```python
from build123d import *

# Parameters (mm, degrees)
SKETCH1_3_W         = 27.034600944
SKETCH1_3_H         = 64.50289226
BOSS_EXTRUDE2_DEPTH = 2
SKETCH1_4_W         = 27.034600944
SKETCH1_4_H         = 64.50289226
SKETCH1_4_R         = 2.5
SKETCH1_4_W_2       = 18.5
SKETCH1_4_H_2       = 23
SKETCH1_4_R_2       = 0.75
BOSS_EXTRUDE3_DEPTH = 3
SKETCH1_R           = 2.5
SKETCH1_R_2         = 0.75
BOSS_EXTRUDE6_DEPTH = 12
CUT_EXTRUDE1_START  = -3
SKETCH2_W           = 10.1
SKETCH2_H           = 7
SKETCH2_H_2         = 5.610263073
CUT_EXTRUDE1_DEPTH  = 3.5
BOSS_EXTRUDE7_DEPTH = 18.5
SKETCH5_W           = 27.034600944
SKETCH5_H           = 64.50289226
SKETCH5_W_2         = 23.034600944
SKETCH5_H_2         = 59.50289226
BOSS_EXTRUDE9_DEPTH = 29
SKETCH6_W           = 23.034600944
SKETCH6_H           = 1
CUT_EXTRUDE2_DEPTH  = 0.5
CUT_EXTRUDE3_REACH  = 75.262
SKETCH8_W           = 14.7
SKETCH8_H           = 8.1
CUT_EXTRUDE4_REACH  = 64.464
SKETCH9_W           = 6.5
SKETCH9_H           = 15.5
SKETCH11_W          = 10.1
SKETCH11_H          = 2
CUT_EXTRUDE5_DEPTH  = 0.5


with BuildPart() as part:
    # Sketch1<3> → Boss-Extrude2 (new body)
    with BuildSketch(Plane.XY):
        with Locations((0, 14.082400554)):
            Rectangle(SKETCH1_3_W, SKETCH1_3_H)
    extrude(amount=BOSS_EXTRUDE2_DEPTH)

    # Sketch1<4> → Boss-Extrude3 (add)
    # profile 1 of 15: a face of its own
    with BuildSketch(Plane.XY):
        with Locations((0, 14.082400554)):
            Rectangle(SKETCH1_4_W, SKETCH1_4_H)
        with Locations((-8.75, -8.667715428)):
            Circle(SKETCH1_4_R, mode=Mode.SUBTRACT)
        with Locations((8.75, -8.667715428)):
            Circle(SKETCH1_4_R, mode=Mode.SUBTRACT)
        with Locations((8.75, 13.832284572)):
            Circle(SKETCH1_4_R, mode=Mode.SUBTRACT)
        with Locations((-8.75, 13.832284572)):
            Circle(SKETCH1_4_R, mode=Mode.SUBTRACT)
        with Locations((0, 32.833846684)):
            Rectangle(SKETCH1_4_W_2, SKETCH1_4_H_2, mode=Mode.SUBTRACT)
    # profile 2 of 15: a face of its own
    with BuildSketch(Plane.XY):
        with Locations((8.75, 13.832284572)):
            Circle(SKETCH1_4_R)
        with Locations((8.75, 13.832284572)):
            Circle(SKETCH1_4_R_2, mode=Mode.SUBTRACT)
    # profile 3 of 15: a face of its own
    with BuildSketch(Plane.XY):
        with Locations((8.75, 13.832284572)):
            Circle(SKETCH1_4_R_2)
    # profile 4 of 15: a face of its own
    with BuildSketch(Plane.XY):
        with Locations((-8.75, 13.832284572)):
            Circle(SKETCH1_4_R)
        with Locations((-8.75, 13.832284572)):
            Circle(SKETCH1_4_R_2, mode=Mode.SUBTRACT)
    # profile 5 of 15: a face of its own
    with BuildSketch(Plane.XY):
        with Locations((-8.75, 13.832284572)):
            Circle(SKETCH1_4_R_2)
    # profile 6 of 15: a face of its own
    with BuildSketch(Plane.XY):
        with BuildLine():
            ThreePointArc((-6.278285008, -8.292715428), (-8.75, -6.167715428), (-11.221714992, -8.292715428))
            Line((-11.221714992, -8.292715428), (-9.399519053, -8.292715428))
            ThreePointArc((-9.399519053, -8.292715428), (-8.75, -7.917715428), (-8.100480947, -8.292715428))
            Line((-8.100480947, -8.292715428), (-6.278285008, -8.292715428))
        make_face()
    # profile 7 of 15: a face of its own
    with BuildSketch(Plane.XY):
        with BuildLine():
            Line((-9.399519053, -8.292715428), (-11.221714992, -8.292715428))
            ThreePointArc((-11.221714992, -8.292715428), (-8.938032605, -11.160634147), (-6.25, -8.667715428))
            ThreePointArc((-6.25, -8.667715428), (-6.257081281, -8.479682824), (-6.278285008, -8.292715428))
            Line((-6.278285008, -8.292715428), (-8.100480947, -8.292715428))
            ThreePointArc((-8.100480947, -8.292715428), (-8.02555563, -8.473601145), (-8, -8.667715428))
            ThreePointArc((-8, -8.667715428), (-8.944114284, -9.392159798), (-9.399519053, -8.292715428))
        make_face()
    # profile 8 of 15: a face of its own
    with BuildSketch(Plane.XY):
        with BuildLine():
            ThreePointArc((-8.100480947, -8.292715428), (-8.75, -7.917715428), (-9.399519053, -8.292715428))
            Line((-9.399519053, -8.292715428), (-8.100480947, -8.292715428))
        make_face()
    # profile 9 of 15: a face of its own
    with BuildSketch(Plane.XY):
        with BuildLine():
            Line((-8.100480947, -8.292715428), (-9.399519053, -8.292715428))
            ThreePointArc((-9.399519053, -8.292715428), (-8.944114284, -9.392159798), (-8, -8.667715428))
            ThreePointArc((-8, -8.667715428), (-8.02555563, -8.473601145), (-8.100480947, -8.292715428))
        make_face()
    # profile 10 of 15: a face of its own
    with BuildSketch(Plane.XY):
        with BuildLine():
            ThreePointArc((-6.278285008, -8.292715428), (-8.75, -6.167715428), (-11.221714992, -8.292715428))
            Line((-11.221714992, -8.292715428), (-9.399519053, -8.292715428))
            ThreePointArc((-9.399519053, -8.292715428), (-8.75, -7.917715428), (-8.100480947, -8.292715428))
            Line((-8.100480947, -8.292715428), (-6.278285008, -8.292715428))
        make_face()
    # profile 11 of 15: a face of its own
    with BuildSketch(Plane.XY):
        with BuildLine():
            Line((-9.399519053, -8.292715428), (-11.221714992, -8.292715428))
            ThreePointArc((-11.221714992, -8.292715428), (-8.938032605, -11.160634147), (-6.25, -8.667715428))
            ThreePointArc((-6.25, -8.667715428), (-6.257081281, -8.479682824), (-6.278285008, -8.292715428))
            Line((-6.278285008, -8.292715428), (-8.100480947, -8.292715428))
            ThreePointArc((-8.100480947, -8.292715428), (-8.02555563, -8.473601145), (-8, -8.667715428))
            ThreePointArc((-8, -8.667715428), (-8.944114284, -9.392159798), (-9.399519053, -8.292715428))
        make_face()
    # profile 12 of 15: a face of its own
    with BuildSketch(Plane.XY):
        with BuildLine():
            ThreePointArc((-8.100480947, -8.292715428), (-8.75, -7.917715428), (-9.399519053, -8.292715428))
            Line((-9.399519053, -8.292715428), (-8.100480947, -8.292715428))
        make_face()
    # profile 13 of 15: a face of its own
    with BuildSketch(Plane.XY):
        with BuildLine():
            Line((-8.100480947, -8.292715428), (-9.399519053, -8.292715428))
            ThreePointArc((-9.399519053, -8.292715428), (-8.944114284, -9.392159798), (-8, -8.667715428))
            ThreePointArc((-8, -8.667715428), (-8.02555563, -8.473601145), (-8.100480947, -8.292715428))
        make_face()
    # profile 14 of 15: a face of its own
    with BuildSketch(Plane.XY):
        with Locations((8.75, -8.667715428)):
            Circle(SKETCH1_4_R)
        with Locations((8.75, -8.667715428)):
            Circle(SKETCH1_4_R_2, mode=Mode.SUBTRACT)
    # profile 15 of 15: a face of its own
    with BuildSketch(Plane.XY):
        with Locations((8.75, -8.667715428)):
            Circle(SKETCH1_4_R_2)
    extrude(amount=-BOSS_EXTRUDE3_DEPTH)

    # Sketch1 → Boss-Extrude6 (add)
    # profile 1 of 4: a face of its own
    with BuildSketch(Plane.XY):
        with BuildLine():
            Line((-9.399519053, -8.292715428), (-11.221714992, -8.292715428))
            ThreePointArc((-11.221714992, -8.292715428), (-8.75, -11.167715428), (-6.278285008, -8.292715428))
            Line((-6.278285008, -8.292715428), (-8.100480947, -8.292715428))
            ThreePointArc((-8.100480947, -8.292715428), (-8.75, -9.417715428), (-9.399519053, -8.292715428))
        make_face()
    # profile 2 of 4: a face of its own
    with BuildSketch(Plane.XY):
        with Locations((-8.75, 13.832284572)):
            Circle(SKETCH1_R)
        with Locations((-8.75, 13.832284572)):
            Circle(SKETCH1_R_2, mode=Mode.SUBTRACT)
    # profile 3 of 4: a face of its own
    with BuildSketch(Plane.XY):
        with Locations((8.75, 13.832284572)):
            Circle(SKETCH1_R)
        with Locations((8.75, 13.832284572)):
            Circle(SKETCH1_R_2, mode=Mode.SUBTRACT)
    # profile 4 of 4: a face of its own
    with BuildSketch(Plane.XY):
        with Locations((8.75, -8.667715428)):
            Circle(SKETCH1_R)
        with Locations((8.75, -8.667715428)):
            Circle(SKETCH1_R_2, mode=Mode.SUBTRACT)
    extrude(amount=-BOSS_EXTRUDE6_DEPTH)

    # Sketch2 → Cut-Extrude1 (cut)
    with BuildSketch(Plane(origin=(0, 0, -3), x_dir=(-1, 0, 0), z_dir=(0, 0, -1)).offset(CUT_EXTRUDE1_START)):
        with Locations((0.3, 40.833846684)):
            Rectangle(SKETCH2_W, SKETCH2_H)
        with Locations((0.3, 47.138978221)):
            Rectangle(SKETCH2_W, SKETCH2_H_2)
    extrude(amount=CUT_EXTRUDE1_DEPTH, mode=Mode.SUBTRACT)

    # Sketch4 → Boss-Extrude7 (add)
    with BuildSketch(Plane.ZY.offset(-9.25)):
        Polygon((-3, 22.333846684), (-3, 21.333846684), (-2.422649731, 21.333846684), align=None)
        Polygon((-3, 20.267009218), (-3, 21.333846684), (-3, 22.333846684), (-4, 21.333846684), (-4, 20.630979452), align=None)
    extrude(amount=BOSS_EXTRUDE7_DEPTH)

    # Sketch5 → Boss-Extrude9 (add)
    with BuildSketch(Plane(origin=(0, 0, -3), x_dir=(-1, 0, 0), z_dir=(0, 0, -1))):
        with Locations((0, 14.082400554)):
            Rectangle(SKETCH5_W, SKETCH5_H)
        with Locations((0, 14.582400554)):
            Rectangle(SKETCH5_W_2, SKETCH5_H_2, mode=Mode.SUBTRACT)
    extrude(amount=BOSS_EXTRUDE9_DEPTH)

    # Sketch6 → Cut-Extrude2 (cut)
    with BuildSketch(Plane(origin=(0, -15.169045576, 0), x_dir=(1, 0, 0), z_dir=(0, 1, 0))):
        with Locations((0, 31)):
            Rectangle(SKETCH6_W, SKETCH6_H)
    extrude(amount=-CUT_EXTRUDE2_DEPTH, mode=Mode.SUBTRACT)

    # Sketch8 → Cut-Extrude3 (cut, up to next)
    with BuildSketch(Plane.XZ.offset(18.169045576), mode=Mode.PRIVATE) as cut_extrude3_sk1:
        with Locations((0, -23.95)):
            Rectangle(SKETCH8_W, SKETCH8_H)
    cut_extrude3_tool1 = extrude(cut_extrude3_sk1.sketch, amount=-CUT_EXTRUDE3_REACH, mode=Mode.PRIVATE) & part.part
    add(cut_extrude3_tool1.solids().sort_by_distance((0, -18.169046, -23.95))[0], mode=Mode.SUBTRACT)

    # Sketch9 → Cut-Extrude4 (cut, up to next)
    with BuildSketch(Plane(origin=(13.517300472, 0, 0), x_dir=(0, 0, -1), z_dir=(1, 0, 0)), mode=Mode.PRIVATE) as cut_extrude4_sk1:
        with Locations((23.75, 14.082400554)):
            Rectangle(SKETCH9_W, SKETCH9_H)
    cut_extrude4_tool1 = extrude(cut_extrude4_sk1.sketch, amount=-CUT_EXTRUDE4_REACH, mode=Mode.PRIVATE) & part.part
    add(cut_extrude4_tool1.solids().sort_by_distance((13.5173, 14.082401, -23.75))[0], mode=Mode.SUBTRACT)

    # Sketch11 → Cut-Extrude5 (cut)
    with BuildSketch(Plane.XY.offset(-3)):
        with Locations((-0.3, 45.333846684)):
            Rectangle(SKETCH11_W, SKETCH11_H)
    extrude(amount=-CUT_EXTRUDE5_DEPTH, mode=Mode.SUBTRACT)


solid = part.part
```
Geometry check sheet. Reference: the model listing, model coordinates, mm. A direction names the side the tool comes from. Round coordinates to 2 decimals unless told otherwise and drop trailing zeros. Write each loop counter-clockwise with the first axis right and the second up, starting at its lowest first coordinate (ties: lowest second). Pieces come first, ordered by that corner, then holes. Notation, with made-up numbers: (29.5, 32) - (79.5, 32) arc R21 ccw to (79.5, 46) - close; hole circle Ø11 at (8.25, 63). An arc over 180 degrees is marked (long way). Write each question's results on one line, items separated by ' | '.
(1) Sectioned sample at D-D, the plane z = -11. Count the separate pieces of the cut face and the enclosed holes in it, plus the area to 3 significant figures.
Computed:
separate pieces: 5 | enclosed holes: 4 | area: 437 mm^2
(2) Depth check by flat-ended pin: pin 1 Ø3 at (x, y) = (-9, 17.5) entering from -Z; pin 2 Ø1.2 at (x, z) = (-4, -1.5) entering from +Y. Enter the tip coordinate at first touch or a pass-through.
Computed:
pin 1: stops at z = -12 | pin 2: stops at y = 21.33
(3) Draft check along X on faces 1 (the face through (0, 15, 2)), 2 (the face through (-13.517, 14, -15)), 3 (the face through (-9, -10, -12)). Enter one of: pulls with the +X half, pulls with the -X half, needs draft (parallel to the pull), parting line crosses it, or undercut.
Computed:
face 1: needs draft | face 2: pulls with the -X half | face 3: undercut
(4) Sectioned sample at A-A, the plane x = 2. Enter the section's corners in (y, z), plus the area to 3 significant figures.
Computed:
outline: (-18.17, -32) - (-15.17, -32) - (-15.17, -31.5) - (-15.67, -31.5) - (-15.67, -30.5) - (-15.17, -30.5) - (-15.17, -28) - (-18.17, -28) - close; (-18.17, -19.9) - (-15.17, -19.9) - (-15.17, -3) - (20.27, -3) - (20.63, -4) - (21.33, -4) - (22.33, -3) - (21.33, -2.42) - (21.33, 0) - (46.33, 0) - (46.33, 2) - (-18.17, 2) - close; (44.33, -32) - (46.33, -32) - (46.33, -3.5) - (44.33, -3.5) - close | area: 368 mm^2
(5) Sectioned sample at B-B, the plane z = -24. Enter the section's corners in (x, y), plus the area to 3 significant figures.
Computed:
outline: (-13.52, -18.17) - (-7.35, -18.17) - (-7.35, -15.17) - (-11.52, -15.17) - (-11.52, 44.33) - (11.52, 44.33) - (11.52, 21.83) - (13.52, 21.83) - (13.52, 46.33) - (-13.52, 46.33) - close; (7.35, -18.17) - (13.52, -18.17) - (13.52, 6.33) - (11.52, 6.33) - (11.52, -15.17) - (7.35, -15.17) - close | area: 298 mm^2
(6) Thickness scan on probe 1 along Y at (x, z) = (8.75, -6.5); probe 2 along Y at (x, z) = (-8.75, -9); probe 3 along X at (y, z) = (29, -23.5). Record the ranges inside material, lowest first. Write a range as from..to.
Computed:
probe 1: y = -18.17..-15.17, -11.17..-9.42, -7.92..-6.17, 11.33..13.08, 14.58..16.33, 44.33..46.33 | probe 2: y = -18.17..-15.17, -11.17..-9.42, 11.33..13.08, 14.58..16.33, 44.33..46.33 | probe 3: x = -13.52..-11.52, 11.52..13.52
(7) Set-up check for faces 4 (the face through (-5.35, 45, -2)), 5 (the face through (-10, -8.293, -7)), 6 (the face through (13, 14, -20.5)): record each of +Z, -Z, +X, -X, +Y, -Y from which the full face is reachable in a straight line by a thin tool's end or side.
Computed:
face 4: +Y | face 5: -Z | face 6: +X
(8) Sectioned sample at C-C, the plane y = 8. Enter the section's corners in (x, z), plus the area to 3 significant figures.
Computed:
outline: (-13.52, -32) - (-11.52, -32) - (-11.52, -3) - (11.52, -3) - (11.52, -20.5) - (13.52, -20.5) - (13.52, 2) - (-13.52, 2) - close; (11.52, -32) - (13.52, -32) - (13.52, -27) - (11.52, -27) - close | area: 238 mm^2
